Autodesk Inventor part; units mm, degrees
ref_plane "YZ Plane" through (0, 0, 0) normal (1, 0, 0) x (0, 1, 0)
ref_plane "XZ Plane" through (0, 0, 0) normal (0, 1, 0) x (-1, 0, 0)
ref_plane "XY Plane" through (0, 0, 0) normal (0, 0, 1) x (1, 0, 0)
sketch "Sketch1" plane through (0, 0, 0) normal (0, 0, 1) x (1, 0, 0)
  circle A0 centre (0, 0) radius 21
  circle A1 centre (16, 0) radius 2
  circle A2 centre (0, 16) radius 2
  circle A3 centre (-16, 0) radius 2
  circle A4 centre (0, -16) radius 2
  line L0 (-14.8492, -14.8492) -> (14.8492, 14.8492)
  line L1 (0, -21) -> (0, 21)
  circle A5 centre (11.3137, 11.3137) radius 1.5
  circle A6 centre (0, 0) radius 12.6
  line L2 (-36.25, -21) -> (36.25, -21)
  line L3 (36.25, 21) -> (-36.25, 21)
  line L4 (-21, -21) -> (21, 21) construction
  line L5 (21, -21) -> (-21, 21) construction
  line L6 (-36.25, 21) -> (-36.25, -21)
  line L7 (36.25, 21) -> (36.25, -21)
  line L8 (-33.35, 17.5) -> (-29.15, 17.5)
  line L9 (-29.15, 17.5) -> (-29.15, -17.5)
  line L10 (-29.15, -17.5) -> (-33.35, -17.5)
  line L11 (-33.35, -17.5) -> (-33.35, 17.5)
  line L12 (-33.35, 17.5) -> (-29.15, -17.5) construction
  line L13 (-29.15, 17.5) -> (-33.35, -17.5) construction
  line L14 (29.15, 17.5) -> (33.35, 17.5)
  line L15 (33.35, 17.5) -> (33.35, -17.5)
  line L16 (33.35, -17.5) -> (29.15, -17.5)
  line L17 (29.15, -17.5) -> (29.15, 17.5)
  line L18 (29.15, 17.5) -> (33.35, -17.5) construction
  line L19 (33.35, 17.5) -> (29.15, -17.5) construction
  line L20 (-26.25, 21) -> (-26.25, -21)
  line L21 (26.25, 21) -> (26.25, -21)
  circle A7 centre (-12.7279, -12.7279) radius 1.621
  circle A8 centre (0, 0) radius 12.5
  circle A9 centre (-12.7279, -12.7279) radius 2
  circle A10 centre (12.7279, 12.7279) radius 2
  circle A11 centre (-12.7279, 12.7279) radius 2
  circle A12 centre (12.7279, -12.7279) radius 2
  circle A13 centre (16, 0) radius 1.6
  circle A14 centre (-16, 0) radius 1.6
  circle A15 centre (0, 16) radius 1.6
  circle A16 centre (0, -16) radius 1.6
  circle A17 centre (0, 0) radius 20.7
  point P0 (-18.984, 8.9782)
  point P1 (-18.984, -8.9782)
  point P2 (-31.25, 0)
  point P3 (31.25, 0)
  point P4 (-31.25, 0)
  point P5 (31.25, 0)
  point P6 (31.25, 0)
  point P7 (31.25, 21)
  point P8 (-31.25, 0)
  point P9 (-31.25, 21)
  point P10 (31.25, 21)
  point P11 (0, 21)
  point P12 (0, -21)
  dimension "d0" = 42
  dimension "d1" = 4
  dimension "d5" = 16
  dimension "d8" = 360
  dimension "d10" = 45
  dimension "d11" = 3
  dimension "d12" = 16
  dimension "d19" = 25.2
  dimension "d31" = 4.2
  dimension "d32" = 35
  dimension "d33" = 4.2
  dimension "d38" = 5
  dimension "d39" = 5
  dimension "d40" = 72.5
  dimension "d41" = 10
  dimension "d42" = 10
extrude "Extrusion1" add sketch "Sketch1" along normal blind 4 contours A0 L1 A17 L0 | A0 L3 L21 L2 | L0 A17 L1 A0 | L2 L20 L3 A0 | A0 L0 A17 L1 | L1 A17 L0 A0 | A17 L1 A4 A6 L0 A5 A10 | L0 A10 A5 A6 L1 A2 A17 | A17 L0 A9 A6 L1 A4 | L2 L6 L3 L20 | L21 L3 L7 L2 | L1 A2 A6 L0 A9 A17 | A10 L0 A5 | A10 A5 L0 picked at (10.8037, 11.1549) picked at (11.1549, 10.8037)
fillet "Fillet1" radius 2 4 edges at (-36.25, 21, 2) (-36.25, -21, 2) (36.25, -21, 2) (36.25, 21, 2)
fillet "Fillet2" radius 2.1 8 edges at (33.35, -17.5, 2) (29.15, -17.5, 2) (29.15, 17.5, 2) (33.35, 17.5, 2) (-33.35, 17.5, 2) (-29.15, 17.5, 2) (-29.15, -17.5, 2) (-33.35, -17.5, 2)
equation "\"d42\" = d41"
properties part number "mounting plate stepper motor base 4 mm" material "Aluminum 6061"
Part model, mm, in its own coordinate system. A direction names the side the tool comes from. Round coordinates to 2 decimals unless told otherwise and drop trailing zeros. Loops run counter-clockwise (first coordinate to the right, second up) from the corner with the lowest first, then second, coordinate; pieces in that order, holes last.
Item 1: Cut at C-C, the plane x = -16. Give the cut face in (y, z).
Item 2: Drop a flat-ended pin along its axis: P1, Ø4.5, axis at x = 12.73, y = -12.73, coming from the +Z side. Give the stop position or say it passes through.
Item 3: Cut at B-B, the plane y = 0. Give the cut face in (x, z).
Item 4: 3-axis set-ups, long thin cutter, end or side, ignore diameter. For faces 1 (the face through (-9, 10, 0)), 2 (the face through (-29.15, 0, 2)): which of +Z, -Z, +X, -X, +Y, -Y reach the whole face in a straight line?
Item 5: Mould opens along X. For faces 3 (the face through (-35.68, -20.4, 2.03)), 4 (the face through (-14.202, 11.376, 1.972)), 5 (the face through (-9, 10, 4)) say: +X half, -X half, draft (parallel to the pull), parting line (faces both ways), or undercut.
Item 6: Cut at A-A, the plane x = 0. Give the cut face in (y, z).
Item 7: Drill centre lines: line 1 (Y direction, x = -16, z = 2.5); line 2 (Y direction, x = 1.5, z = 3.35); line 3 (X direction, y = 4.5, z = 2.6). Where is each one in solid material? Low to high.
Item 8: Cut at D-D, the plane y = 9.5. Give the cut face in (x, z), then the cut area to 3 significant figures.
A:
1. outline: (-21, 0) - (-2, 0) - (-2, 4) - (-21, 4) - close; (2, 0) - (21, 0) - (21, 4) - (2, 4) - close
2. P1: stops at z = 4
3. outline: (-36.25, 0) - (-33.35, 0) - (-33.35, 4) - (-36.25, 4) - close; (-29.15, 0) - (-18, 0) - (-18, 4) - (-29.15, 4) - close; (-14, 0) - (-12.6, 0) - (-12.6, 4) - (-14, 4) - close; (12.6, 0) - (14, 0) - (14, 4) - (12.6, 4) - close; (18, 0) - (29.15, 0) - (29.15, 4) - (18, 4) - close; (33.35, 0) - (36.25, 0) - (36.25, 4) - (33.35, 4) - close
4. face 1: -Z, +X, -X, +Y, -Y
4. face 2: +Z, -Z
5. face 3: -X half
5. face 4: undercut
5. face 5: draft
6. outline: (-21, 0) - (-18, 0) - (-18, 4) - (-21, 4) - close; (-14, 0) - (-12.6, 0) - (-12.6, 4) - (-14, 4) - close; (12.6, 0) - (14, 0) - (14, 4) - (12.6, 4) - close; (18, 0) - (21, 0) - (21, 4) - (18, 4) - close
7. line 1: y = -21 to -2, 2 to 21
7. line 2: y = -21 to -17.32, -14.68 to -12.51, 12.51 to 14.68, 17.32 to 21
7. line 3: x = -36.25 to -33.35, -29.15 to -11.77, 11.77 to 29.15, 33.35 to 36.25
8. outline: (-36.25, 0) - (-33.35, 0) - (-33.35, 4) - (-36.25, 4) - close; (-29.15, 0) - (-8.28, 0) - (-8.28, 4) - (-29.15, 4) - close; (8.28, 0) - (29.15, 0) - (29.15, 4) - (8.28, 4) - close; (33.35, 0) - (36.25, 0) - (36.25, 4) - (33.35, 4) - close
8. area: 190 mm2
